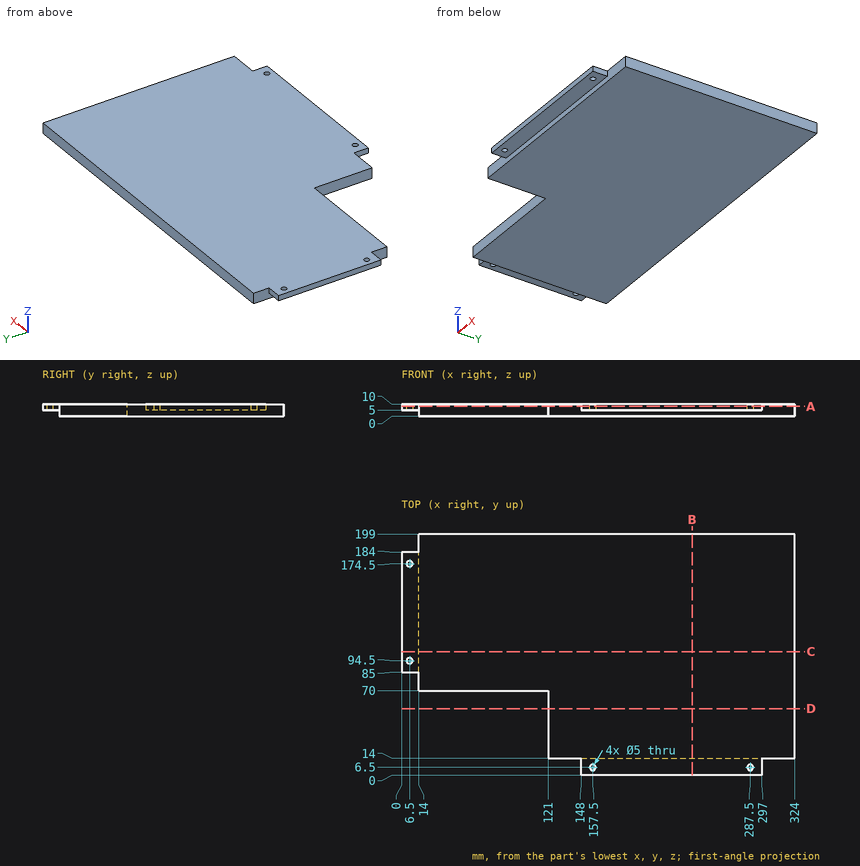
Can you work these out from the drawing? Everything is in mm from the part's minimum corner. Coordinates: 2 decimals unless noted, no trailing zeros. Loops run counter-clockwise (first coordinate to the right, second up) from the corner with the lowest first, then second, coordinate; pieces in that order, holes last. Notation, with made-up numbers: M -7.5,21.5 L 2.5,21.5 A22 cw 2.5,52.5 Z; hole C 62.25,38.5 d10. An arc over 180 degrees is marked long. Put each result on its own line as item: value. Start each with the question number.
(1) Suppose I cut it at C-C on y = 102. Please give me the cut outline in (x, z).
(2) Will these pins go through, and if not, where does the flat tip stop? P1, Ø3, axis at y = 54, z = 7.5, coming from the -X side; P2, Ø11, axis at x = 7, y = 111, coming from the -Z side; P3, Ø4, axis at y = 4.5, z = 7.5, coming from the -X side; P4, Ø4, axis at x = 287.5, y = 6.5, coming from the +Z side.
(3) Suppose I cut it at B-B on x = 239.5. Please give me the cut outline in (y, z), then the cut area to 3 significant figures.
(4) Suppose I cut it at A-A on z = 8. Please give me the cut outline in (x, y).
(5) I need wall thicknesses on line 1 (Y direction, x = 6.5, z = 6.7); line 2 (Y direction, x = 157.5, z = 9.05); line 3 (X direction, y = 174.5, z = 6). Which ranges of each line are inside material? Lowest first, please. Write a range as from..to.
(6) Suppose I cut it at D-D on y = 55. Please give me the cut outline in (x, z), then the cut area to 3 significant figures.
Solutions:
1. outline: M 0,5 L 14,5 L 14,0 L 324,0 L 324,10 L 0,10 Z
2. P1: stops at x = 121
2. P2: stops at z = 5
2. P3: stops at x = 148
2. P4: passes through
3. outline: M 0,5 L 14,5 L 14,0 L 199,0 L 199,10 L 0,10 Z
3. area: 1,920 mm2
4. outline: M 0,85 L 14,85 L 14,70 L 121,70 L 121,14 L 148,14 L 148,0 L 297,0 L 297,14 L 324,14 L 324,199 L 14,199 L 14,184 L 0,184 Z; hole C 6.5,94.5 d5; hole C 6.5,174.5 d5; hole C 157.5,6.5 d5; hole C 287.5,6.5 d5
5. line 1: y = 85..92, 97..172, 177..184
5. line 2: y = 0..4, 9..199
5. line 3: x = 0..4, 9..324
6. outline: M 121,0 L 324,0 L 324,10 L 121,10 Z
6. area: 2,030 mm2
